Source: CAD feature listing. Evaluate the final solid. Frame: model axes, mm. Round coordinates to 2 decimals unless told otherwise and drop trailing zeros. Loops run counter-clockwise (first coordinate to the right, second up) from the corner with the lowest first, then second, coordinate; pieces in that order, holes last. Notation, with made-up numbers: (76.5, -22) - (124.5, -22) arc R18 ccw to (124.5, 8) - close; hole circle Ø3 at (51, -15.75). An arc over 180 degrees is marked (long way). Write item = value, one per line. Start each with the question number.
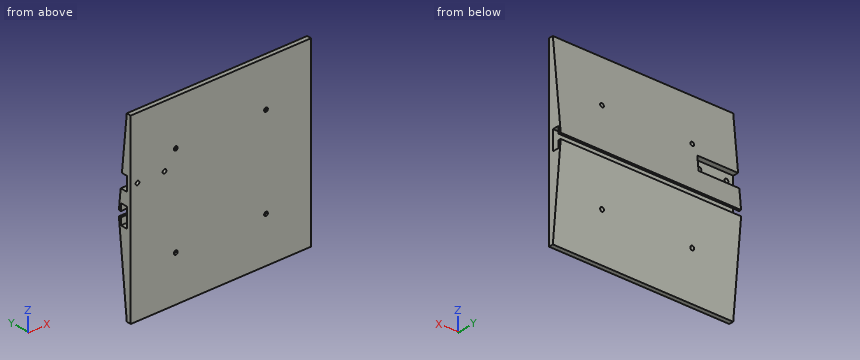
from build123d import *

# Parameters (mm, degrees)
SKETCH1_W           = 200
SKETCH1_H           = 200
BOSS_EXTRUDE1_DEPTH = 5
BOSS_EXTRUDE2_DEPTH = 200
CUT_EXTRUDE9_START  = -200
SKETCH13_W          = 21.4
SKETCH13_H          = 7.5
CUT_EXTRUDE9_DEPTH  = 200
CUT_EXTRUDE14_START = -2
CUT_EXTRUDE14_DEPTH = 3.6
SKETCH17_R          = 2.1
CUT_EXTRUDE15_DEPTH = 16
SKETCH19_W          = 15.4
SKETCH19_H          = 7.75257732
CUT_EXTRUDE16_DEPTH = 45.2
SKETCH20_R          = 2.1
CUT_EXTRUDE17_DEPTH = 45


with BuildPart() as part:
    # Sketch1 → Boss-Extrude1 (new body)
    with BuildSketch(Plane(origin=(0, 0, 0), x_dir=(1, 0, 0), z_dir=(0, 1, 0))):
        Rectangle(SKETCH1_W, SKETCH1_H)
    extrude(amount=BOSS_EXTRUDE1_DEPTH)

    # Sketch9 → Boss-Extrude2 (add)
    with BuildSketch(Plane(origin=(100, 0, 0), x_dir=(0, 0, -1), z_dir=(1, 0, 0))):
        Polygon((-100, 5), (-3, 15), (-3, 5), align=None)
        Polygon((3, 5), (100, 5), (3, 15), align=None)
    extrude(amount=-BOSS_EXTRUDE2_DEPTH)

    # Sketch13 → Cut-Extrude9 (cut)
    with BuildSketch(Plane.ZY.offset(100).offset(CUT_EXTRUDE9_START)):
        with Locations((0, 8.75)):
            Rectangle(SKETCH13_W, SKETCH13_H)
    extrude(amount=CUT_EXTRUDE9_DEPTH, mode=Mode.SUBTRACT)

    # Sketch18 → Cut-Extrude14 (cut)
    with BuildSketch(Plane.XZ.offset(CUT_EXTRUDE14_START)):
        Polygon((-52.136195996, 46.3), (-47.863804004, 46.3), (-45.727608008, 50), (-47.863804004, 53.7), (-52.136195996, 53.7), (-54.272391992, 53.7), (-54.272391992, 46.3), align=None)
        Polygon((47.863804004, 46.3), (52.136195996, 46.3), (54.272391992, 50), (52.136195996, 53.7), (47.863804004, 53.7), (45.727608008, 53.7), (45.727608008, 46.3), align=None)
        Polygon((47.863804004, -53.7), (52.136195996, -53.7), (54.272391992, -50), (52.136195996, -46.3), (47.863804004, -46.3), (45.727608008, -46.3), (45.727608008, -53.7), align=None)
        Polygon((-52.136195996, -53.7), (-47.863804004, -53.7), (-45.727608008, -50), (-47.863804004, -46.3), (-52.136195996, -46.3), (-54.272391992, -46.3), (-54.272391992, -53.7), align=None)
    extrude(amount=-CUT_EXTRUDE14_DEPTH, mode=Mode.SUBTRACT)

    # Sketch17 → Cut-Extrude15 (cut, through all)
    with BuildSketch(Plane.XZ):
        with Locations((-50, 50)):
            Circle(SKETCH17_R)
        with Locations((50, 50)):
            Circle(SKETCH17_R)
        with Locations((50, -50)):
            Circle(SKETCH17_R)
        with Locations((-50, -50)):
            Circle(SKETCH17_R)
    extrude(amount=-CUT_EXTRUDE15_DEPTH, mode=Mode.SUBTRACT)

    # Sketch19 → Cut-Extrude16 (cut)
    with BuildSketch(Plane.ZY.offset(100)):
        with Locations((32.5, 8.87628866)):
            Rectangle(SKETCH19_W, SKETCH19_H)
    extrude(amount=-CUT_EXTRUDE16_DEPTH, mode=Mode.SUBTRACT)

    # Sketch20 → Cut-Extrude17 (cut)
    with BuildSketch(Plane(origin=(0, 5, 0), x_dir=(1, 0, 0), z_dir=(0, 1, 0))):
        with Locations((-92.5, -32.5)):
            Circle(SKETCH20_R)
        with Locations((-62.5, -32.5)):
            Circle(SKETCH20_R)
    extrude(amount=-CUT_EXTRUDE17_DEPTH, mode=Mode.SUBTRACT)


solid = part.part
(1) Material intervals for line 1 along X through (y, z) = (8.4, -50); line 2 along X through (y, z) = (4.75, 50); line 3 along Y through (x, z) = (-72.5, -6.5), sorted ascending. Write a range as from..to.
(2) Pin query (flat end, axial travel): P1, Ø5, axis at x = -50, z = 50, coming from the +Y side; P2, Ø17, axis at x = -66.5, z = 32, coming from the +Y side; P3, Ø2, axis at x = -23.5, z = 17.5, coming from the -Y side; P4, Ø4, axis at x = -36, z = -67, coming from the +Y side. Return the tip coordinate at first contact, or that it passes through.
(3) Cut plane D-D (z = -81). Output: boundary loops of the cut face in (x, y), and give its area (3 significant figures).
(4) Cut plane A-A (x = 79). Output: boundary loops of the cut face in (y, z).
(5) Cut plane C-C (z = -30). Output: boundary loops of the cut face in (x, y), and give its area (3 significant figures).
(6) Cut plane B-B (z = -7). Output: boundary loops of the cut face in (x, y), and give its area (3 significant figures).
Solution:
q1.line_1 = -100..-52.1, -47.9..47.9, 52.1..100
q1.line_2 = -100..-54.27, -45.73..45.73, 54.27..100
q1.line_3 = 0..5, 12.5..14.64
q2.P1 = 10.41
q2.P2 = 12.89
q2.P3 = 0
q2.P4 = 8.61
q3.outline = (-100, 0) - (100, 0) - (100, 6.96) - (-100, 6.96) - close
q3.area = 1,390 mm^2
q4.outline = (0, -100) - (5, -100) - (15, -3) - (12.5, -3) - (12.5, -10.7) - (5, -10.7) - (5, 10.7) - (12.5, 10.7) - (12.5, 3) - (15, 3) - (5, 100) - (0, 100) - close
q5.outline = (-100, 0) - (100, 0) - (100, 12.22) - (-100, 12.22) - close
q5.area = 2,440 mm^2
q6.outline = (-100, 0) - (100, 0) - (100, 5) - (-100, 5) - close; (-100, 12.5) - (100, 12.5) - (100, 14.59) - (-100, 14.59) - close
q6.area = 1,420 mm^2
